The model under review builds one solid part; all positions refer to its coordinate system, in mm. Face numbers are marked on the shaded views. A direction names the side the tool comes from. Round coordinates to 2 decimals unless told otherwise and drop trailing zeros. Write each loop counter-clockwise with the first axis right and the second up, starting at its lowest first coordinate (ties: lowest second). Pieces come first, ordered by that corner, then holes. Notation, with made-up numbers: (89, -18.5) -> (112, -18.5) arc R4 ccw to (112, -11.5) -> close; hole circle Ø1 at (-17.75, 59). An arc over 180 degrees is marked (long way). Answer in a Markdown table with one row per item. Add a question column.
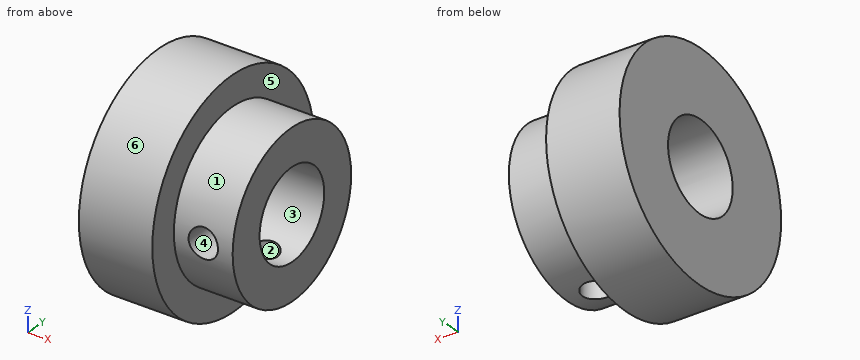
```python
from build123d import *

# Parameters (mm, degrees)
SCHIZZO2_R               = 2
TAGLIO_ESTRUSIONE1_DEPTH = 33.921195442
SCHIZZO3_R               = 2
TAGLIO_ESTRUSIONE2_DEPTH = 33.921195518


with BuildPart() as part:
    # Schizzo1 → Rivoluzione1 (revolve)
    with BuildSketch(Plane.XY, mode=Mode.PRIVATE) as rivoluzione1_sk:
        Polygon((-25.175486278, 6), (-25.175486278, 15), (-15.175486278, 15), (-15.175486278, 11), (-7.175486278, 11), (-7.175486278, 6), align=None)
    revolve(rivoluzione1_sk.sketch.rotate(Axis((88.99, 0, 0), (-1, 0, 0)), 90), axis=Axis((88.99, 0, 0), (-1, 0, 0)))

    # Schizzo2 → Taglio-Estrusione1 (cut, through all)
    with BuildSketch(Plane.XY):
        with Locations((-11.175486278, 0)):
            Circle(SCHIZZO2_R)
    extrude(amount=-TAGLIO_ESTRUSIONE1_DEPTH, mode=Mode.SUBTRACT)

    # Schizzo3 → Taglio-Estrusione2 (cut, through all)
    with BuildSketch(Plane(origin=(0, 0, 0), x_dir=(1, 0, 0), z_dir=(0, 1, 0))):
        with Locations(Location((-11.175486278, 0, 0), (0, 0, 270))):
            Circle(SCHIZZO3_R)
    extrude(amount=-TAGLIO_ESTRUSIONE2_DEPTH, mode=Mode.SUBTRACT)


solid = part.part
```
1. Insertion check: pin 1 Ø3.5 at (x, z) = (-11.18, 0) entering from +Y; pin 2 Ø1 at (y, z) = (2, 3) entering from +X; pin 3 Ø1.5 at (x, z) = (-20, -11.5) entering from +Y; pin 4 Ø2 at (x, y) = (-21.5, -9) entering from -Z. Each pin has a flat end and moves straight along its axis. Give the tip position at first contact, or say it passes through.
2. Add section C-C on x = -20.5. Write out the cut boundary in (y, z), plus the area to 3 significant figures.
3. Tool access review of the marked faces 1, 2 and 3: name each direction out of +Z, -Z, +X, -X, +Y, -Y from which nothing blocks a thin tool from reaching the whole face with its end or side.
4. Add section D-D on z = 7. Write out the cut boundary in (x, y).
5. For L1, parallel to Y at x = -16.75, z = 0; L2, parallel to X at y = -7.75, z = 0; L3, parallel to Y at x = -13.5, z = -1.5, list the stretches that pass through material, from the lowest coordinate up.
6. Add section A-A on y = 0. Write out the cut boundary in (x, z), plus the area to 3 significant figures.
7. Mouldability with a two-part tool opening along Z and no side actions: class the marked faces 4, 5 and 6 as pulls with the +Z half, pulls with the -Z half, needs draft (parallel to the pull), parting line crosses it, or undercut.
Filled in:
| question | item | result |
|---|---|---|
| 1 | pin 1 | y = 11 |
| 1 | pin 2 | through |
| 1 | pin 3 | y = 10.46 |
| 1 | pin 4 | z = -12.69 |
| 2 | outline | circle Ø30 at (0, 0); hole circle Ø12 at (0, 0) |
| 2 | area | 594 mm² |
| 3 | face 1 | +X |
| 3 | face 2 | -Z |
| 3 | face 3 | +X, -X |
| 4 | outline | (-25.18, -13.27) -> (-15.18, -13.27) -> (-15.18, -8.49) -> (-7.18, -8.49) -> (-7.18, 8.49) -> (-15.18, 8.49) -> (-15.18, 13.27) -> (-25.18, 13.27) -> close |
| 5 | L1 | -15 to -6, 6 to 15 |
| 5 | L2 | -25.18 to -13.18, -9.18 to -7.18 |
| 5 | L3 | -10.9 to -5.81, 5.81 to 10.9 |
| 6 | outline | (-25.18, -15) -> (-15.18, -15) -> (-15.18, -11) -> (-13.18, -11) -> (-13.18, -6) -> (-25.18, -6) -> close; (-25.18, 6) -> (-7.18, 6) -> (-7.18, 11) -> (-15.18, 11) -> (-15.18, 15) -> (-25.18, 15) -> close; (-9.18, -11) -> (-7.18, -11) -> (-7.18, -6) -> (-9.18, -6) -> close |
| 6 | area | 240 mm² |
| 7 | face 4 | undercut |
| 7 | face 5 | needs draft |
| 7 | face 6 | parting line crosses it |
